Could you check a few things on this model? Use its own coordinates, in mm. A direction names the side the tool comes from. Round coordinates to 2 decimals unless told otherwise and drop trailing zeros. Loops run counter-clockwise (first coordinate to the right, second up) from the corner with the lowest first, then second, coordinate; pieces in that order, holes last. Notation, with made-up numbers: M 69,16 L 92,16 A21 cw 92,41 Z; hole C 42.25,-5.75 d5. An arc over 180 degrees is marked long. One line per item, written item: value. Start each with the question number.
Q1. Imagine slicing it at C-C (y = 14). Please give me the cut outline in (x, z).
Q2. Imagine slicing it at B-B (y = 0). Please give me the cut outline in (x, z) (3 decimals), then the cut area to 3 significant figures.
Q3. Which directions (+Z, -Z, +X, -X, +Y, -Y) give clear straight access to the entire face, cutting with the end or side of a thin tool? Please do faces 1 (the face through (0, 22, -2)), 2 (the face through (-4, 22.3, 0.7)), 3 (the face through (4, 23, 1)).
Q4. Imagine slicing it at D-D (z = -0.5). Please give me the cut outline in (x, y), then the cut area to 3 significant figures.
Q5. Thinking about a two-plate mould opening in Y: for faces 4 (the face through (-2, 4, 0)), 5 (the face through (-3.2, -1.7, 2.5)), 6 (the face through (3, -4, 2)), 7 (the face through (0, 30, -1)), which applies, released by +Y, released by -Y, zero draft, split by the parting line, or undercut?
Q6. Imagine slicing it at A-A (x = 0). Please give me the cut outline in (y, z) (3 decimals), then the cut area to 3 significant figures.
Q7. I'm going to push flat-ended pins straight in: pin 1 Ø4 at (x, y) = (1.5, 8) entering from -Z; pin 2 Ø5 at (x, z) = (0.5, -3) entering from -Y; pin 3 Ø2 at (x, z) = (-1.5, 0.5) entering from -Y; pin 4 Ø3 at (x, y) = (0.5, 0) entering from -Z. Where does each tip first touch, or does it pass through?
Q8. Please list where these lines run through material, in increasing order: line 1 along X through (y, z) = (0, 1.4) (3 decimals); line 2 along Z through (x, y) = (-1.75, 21.5); line 3 along Y through (x, z) = (-1.5, -2.5).
Solid Edge part; units mm, degrees
sketch "Sketch1" plane through (0, 0, 0) normal (0, 0, 1) x (1, 0, 0)
  circle A0 centre (0, 0) radius 2.5
  circle A1 centre (0, 0) radius 5
extrude "Protrusion1" add sketch "Sketch1" along normal blind 5
sketch "Sketch2" plane through (0, 0, 5) normal (0, 0, 1) x (1, 0, 0)
  line L0 (-4, 3) -> (4, 3)
  line L1 (4, 30) -> (4, 3)
  line L2 (-4, 30) -> (4, 30)
  line L3 (-4, 3) -> (-4, 30)
  dimension "D1" = 4
extrude "ExtrudedProtrusion_2" add sketch "Sketch2" against normal blind 3
sketch "Sketch3" plane through (0, 16.5, 2) normal (0, 0, -1) x (0, 1, 0)
  line L0 (13.5, 4) -> (13.5, -4)
  line L1 (13.5, -4) -> (5.5, -4)
  line L2 (5.5, -4) -> (5.5, 4)
  line L3 (5.5, 4) -> (13.5, 4)
  dimension "D1" = 5.5
extrude "ExtrudedProtrusion_3" add sketch "Sketch3" along normal blind 8.35
hole "Hole_1" at (0, 0, 5) direction (0, 0, -1) diameter 7.25 end up to next start chamfer 0.6 start chamfer angle 45 end chamfer 0.6 end chamfer angle 45
properties material "Polyethylene, low density"
Report:
1. outline: M -4,2 L 4,2 L 4,5 L -4,5 Z
2. outline: M -5,0 L -4.225,0 L -3.625,0.6 L -3.625,4.4 L -4.225,5 L -5,5 Z; M 3.625,0.6 L 4.225,0 L 5,0 L 5,5 L 4.225,5 L 3.625,4.4 Z
2. area: 13.0 mm²
3. face 1: -Z, +X, -X
3. face 2: +Z, -Z, -X, +Y
3. face 3: +Z, -Z, +X, +Y
4. outline: M -4,22 L 4,22 L 4,30 L -4,30 Z
4. area: 64.0 mm²
5. face 4: zero draft
5. face 5: undercut
5. face 6: undercut
5. face 7: released by +Y
6. outline: M -5,0 L -4.225,0 L -3.625,0.6 L -3.625,4.4 L -4.225,5 L -5,5 Z; M 3.625,0.6 L 4.225,0 L 5,0 L 5,2 L 22,2 L 22,-6.35 L 30,-6.35 L 30,5 L 4.225,5 L 3.625,4.4 Z
6. area: 155 mm²
7. pin 1: stops at z = 2
7. pin 2: stops at y = 22
7. pin 3: stops at y = -4.97
7. pin 4: passes through
8. line 1: x = -5 to -3.625, 3.625 to 5
8. line 2: z = 2 to 5
8. line 3: y = 22 to 30
